Read the model definition and answer for the solid it produces. Units are mm, in the model's axes. A direction names the side the tool comes from. Give positions to 0.01 mm unless a question says otherwise; leave off trailing zeros. Loops run counter-clockwise (first coordinate to the right, second up) from the corner with the lowest first, then second, coordinate; pieces in that order, holes last.
(1) Which of the six approach directions +Z, -Z, +X, -X, +Y, -Y give full straight-line access (tool end or side, diameter ignored) to faces 1 (the face through (31.1, 9, 3)), 2 (the face through (47, 2.05, 6)), 3 (the face through (38, 5, 3.75)), 4 (the face through (59, 9.4, 6)), 5 (the face through (44.2, 4, 6))?
(2) Each of these flat-tipped pins is pushed along its axis until it touches: P1, Ø5, axis at x = 34.5, y = 8, coming from the -Z side; P2, Ø1.4, axis at x = 47, y = 3.5, coming from the +Z side; P3, Ø4.5, axis at x = 54.5, z = 8, coming from the +Y side; P4, Ø6, axis at y = 5, z = 6.5, coming from the -X side. Where does it stop, or does it pass through?
(3) Determine the mould class of faces 6 (the face through (39, 9, 5)), 7 (the face through (30, 8.9, -2)) for opening direction X: pulls with the +X half, pulls with the -X half, needs draft (parallel to the pull), parting line crosses it, or undercut.
(4) Straight lines are drawn through the part: probe 1 along X at (y, z) = (8.95, 6); probe 2 along X at (y, z) = (9.5, 3.75); probe 3 along Z at (x, y) = (32, 7.75). For each, find the intervals that lie inside material, in ascending order.
(5) Find section A-A, the plane x = 19. Write down the section's boundary in (y, z), then the cut area to 3 significant figures.
```python
from build123d import *
from build123d.topology import SkipClean

# Parameters (mm, degrees)
CROQUIS1_W              = 60.9
CROQUIS1_H              = 12
SALIENTE_EXTRUIR1_DEPTH = 14
CROQUIS2_OUTSIDE_W      = 75.626
CROQUIS2_OUTSIDE_H      = 26.726
CROQUIS2_OUTSIDE_R      = 1.5
CORTAR_EXTRUIR1_DEPTH   = 4
SALIENTE_EXTRUIR3_DEPTH = 1.1
CROQUIS4_OUTSIDE_W      = 75.752
CROQUIS4_OUTSIDE_H      = 29.852
CORTAR_EXTRUIR2_DEPTH   = 0.7
CORTAR_EXTRUIR3_DEPTH   = 2.5
CROQUIS6_W              = 1.45
CROQUIS6_H              = 3.1
CROQUIS6_W_2            = 1
CORTAR_EXTRUIR4_DEPTH   = 0.1
REDONDEO1_R             = 1
REDONDEO2_R             = 1
SALIENTE_EXTRUIR4_DEPTH = 0.1
CORTAR_EXTRUIR5_REACH   = 64.764
CROQUIS8_R              = 1.15
CROQUIS9_OUTSIDE_W      = 75.752
CROQUIS9_OUTSIDE_H      = 29.852
CORTAR_EXTRUIR7_DEPTH   = 5.55
SALIENTE_EXTRUIR6_DEPTH = 3.5
CROQUIS12_W             = 31.6
CROQUIS12_H             = 1.3
CORTAR_EXTRUIR8_DEPTH   = 2.3
CROQUIS14_W             = 1.3
CROQUIS14_H             = 1
CORTAR_EXTRUIR9_DEPTH   = 2.3
REDONDEO3_R             = 1
CROQUIS15_W             = 7.62
CROQUIS15_H             = 9.4
CROQUIS15_W_2           = 7.6
CORTAR_EXTRUIR10_DEPTH  = 1.9
REDONDEO4_R             = 1.3
REDONDEO5_R             = 1.3
REDONDEO6_R             = 1.3
REDONDEO7_R             = 1


# Some blends are built 0.0001 mm under size
with BuildPart() as part:
    # Croquis1 → Saliente-Extruir1 (new body)
    with BuildSketch(Plane(origin=(0, 0, 0), x_dir=(1, 0, 0), z_dir=(0, 1, 0))):
        with Locations((30.45, -6)):
            Rectangle(CROQUIS1_W, CROQUIS1_H)
    extrude(amount=SALIENTE_EXTRUIR1_DEPTH)

    # Croquis2 outside → Cortar-Extruir1 (cut)
    with BuildSketch(Plane(origin=(0, 14, 0), x_dir=(1, 0, 0), z_dir=(0, 1, 0))):
        with Locations((30.45, -6)):
            Rectangle(CROQUIS2_OUTSIDE_W, CROQUIS2_OUTSIDE_H)
        with Locations(Location((30.45, -6, 0), (0, 0, 270))):
            Circle(CROQUIS2_OUTSIDE_R, mode=Mode.SUBTRACT)
    extrude(amount=-CORTAR_EXTRUIR1_DEPTH, mode=Mode.SUBTRACT)

    # Croquis3 → Saliente-Extruir3 (add)
    with BuildSketch(Plane(origin=(0, 10, 0), x_dir=(1, 0, 0), z_dir=(0, 1, 0))):
        Polygon((30.45, 0), (29.45, 0), (29.45, 3), (31.45, 3), (31.45, 0), align=None)
    extrude(amount=-SALIENTE_EXTRUIR3_DEPTH)

    # Croquis4 outside → Cortar-Extruir2 (cut)
    with BuildSketch(Plane(origin=(0, 10, 0), x_dir=(1, 0, 0), z_dir=(0, 1, 0))):
        with Locations((30.45, -4.5)):
            Rectangle(CROQUIS4_OUTSIDE_W, CROQUIS4_OUTSIDE_H)
        Polygon((8.9, -6), (8.9, 0), (29.45, 0), (29.45, 3), (31.45, 3), (31.45, 0), (52, 0), (52, -12), (8.9, -12), align=None, mode=Mode.SUBTRACT)
    extrude(amount=-CORTAR_EXTRUIR2_DEPTH, mode=Mode.SUBTRACT)

    # Croquis5 → Cortar-Extruir3 (cut)
    with SkipClean():  # the faces are left unmerged after this step: merging them gives an invalid solid
        with BuildSketch(Plane(origin=(0, 10, 0), x_dir=(1, 0, 0), z_dir=(0, 1, 0))):
            with BuildLine():
                ThreePointArc((29.331966011, -5), (29.548647819, -4.801015327), (29.8, -4.648149417))
                Line((29.8, -4.648149417), (29.8, -1.9))
                Line((29.8, -1.9), (11.4, -1.9))
                Line((11.4, -1.9), (11.4, -5))
                Line((11.4, -5), (29.331966011, -5))
            make_face()
            with BuildLine():
                ThreePointArc((29.8, -7.351850583), (29.548647819, -7.198984673), (29.331966011, -7))
                Line((29.331966011, -7), (11.4, -7))
                Line((11.4, -7), (11.4, -10.1))
                Line((11.4, -10.1), (29.8, -10.1))
                Line((29.8, -10.1), (29.8, -7.351850583))
            make_face()
            with BuildLine():
                Line((49.05, -7), (31.568033989, -7))
                ThreePointArc((31.568033989, -7), (31.351352181, -7.198984673), (31.1, -7.351850583))
                Line((31.1, -7.351850583), (31.1, -10.1))
                Line((31.1, -10.1), (49.05, -10.1))
                Line((49.05, -10.1), (49.05, -7))
            make_face()
            with BuildLine():
                Line((49.05, -5), (49.05, -1.9))
                Line((49.05, -1.9), (31.1, -1.9))
                Line((31.1, -1.9), (31.1, -4.648149417))
                ThreePointArc((31.1, -4.648149417), (31.351352181, -4.801015327), (31.568033989, -5))
                Line((31.568033989, -5), (49.05, -5))
            make_face()
        extrude(amount=-CORTAR_EXTRUIR3_DEPTH, mode=Mode.SUBTRACT)

    # Croquis6 → Cortar-Extruir4 (cut)
    with SkipClean():  # the faces are left unmerged after this step: merging them gives an invalid solid
        with BuildSketch(Plane(origin=(0, 10, 0), x_dir=(1, 0, 0), z_dir=(0, 1, 0))):
            with Locations((49.775, -3.45)):
                Rectangle(CROQUIS6_W, CROQUIS6_H)
            with Locations((49.55, -8.55)):
                Rectangle(CROQUIS6_W_2, CROQUIS6_H)
            with Locations((10.9, -3.45)):
                Rectangle(CROQUIS6_W_2, CROQUIS6_H)
            with Locations((10.9, -8.55)):
                Rectangle(CROQUIS6_W_2, CROQUIS6_H)
        extrude(amount=-CORTAR_EXTRUIR4_DEPTH, mode=Mode.SUBTRACT)

    # Redondeo1
    redondeo1_edges = [part.edges().sort_by_distance(p)[0] for p in [
        (31.45, 9.45, -3),
    ]]
    fillet(redondeo1_edges, radius=REDONDEO1_R)

    # Redondeo2
    redondeo2_edges = [part.edges().sort_by_distance(p)[0] for p in [
        (29.45, 9.45, -3),
    ]]
    fillet(redondeo2_edges, radius=REDONDEO2_R - 0.0001)  # a hair under: the kernel refuses the full size

    # Croquis7 → Saliente-Extruir4 (add)
    with BuildSketch(Plane(origin=(0, 9.3, 0), x_dir=(1, 0, 0), z_dir=(0, 1, 0))):
        with BuildLine():
            Line((57.45, -8.8), (57.45, -7.15))
            ThreePointArc((57.45, -7.15), (58.6, -6), (57.45, -4.85))
            Line((57.45, -4.85), (57.45, -3.2))
            ThreePointArc((57.45, -3.2), (60.25, -6), (57.45, -8.8))
        make_face()
        with BuildLine():
            Line((3.75, -4.85), (3.75, -3.2))
            ThreePointArc((3.75, -3.2), (0.95, -6), (3.75, -8.8))
            Line((3.75, -8.8), (3.75, -7.15))
            ThreePointArc((3.75, -7.15), (2.6, -6), (3.75, -4.85))
        make_face()
    extrude(amount=SALIENTE_EXTRUIR4_DEPTH)

    # Croquis8 → Cortar-Extruir5 (cut, up to next)
    with BuildSketch(Plane(origin=(0, 9.3, 0), x_dir=(1, 0, 0), z_dir=(0, 1, 0)), mode=Mode.PRIVATE) as cortar_extruir5_sk1:
        with Locations(Location((57.45, -6, 0), (0, 0, 90))):
            Circle(CROQUIS8_R)
    cortar_extruir5_tool1 = extrude(cortar_extruir5_sk1.sketch, amount=-CORTAR_EXTRUIR5_REACH, mode=Mode.PRIVATE) & part.part
    # Croquis8 → Cortar-Extruir5 (cut, up to next)
    with BuildSketch(Plane(origin=(0, 9.3, 0), x_dir=(1, 0, 0), z_dir=(0, 1, 0)), mode=Mode.PRIVATE) as cortar_extruir5_sk2:
        with Locations(Location((3.75, -6, 0), (0, 0, 90))):
            Circle(CROQUIS8_R)
    cortar_extruir5_tool2 = extrude(cortar_extruir5_sk2.sketch, amount=-CORTAR_EXTRUIR5_REACH, mode=Mode.PRIVATE) & part.part
    add(cortar_extruir5_tool1.solids().sort_by_distance((57.45, 9.3, 6))[0], mode=Mode.SUBTRACT)
    add(cortar_extruir5_tool2.solids().sort_by_distance((3.75, 9.3, 6))[0], mode=Mode.SUBTRACT)

    # Croquis9 outside → Cortar-Extruir7 (cut)
    with BuildSketch(Plane.XZ):
        with Locations((30.45, 4.5)):
            Rectangle(CROQUIS9_OUTSIDE_W, CROQUIS9_OUTSIDE_H)
        Polygon((30, 7.25), (28.1, 7.25), (28.1, 4.75), (31.9, 4.75), (31.9, 7.25), align=None, mode=Mode.SUBTRACT)
    extrude(amount=-CORTAR_EXTRUIR7_DEPTH, mode=Mode.SUBTRACT)

    # Croquis10 → Saliente-Extruir6 (add)
    with BuildSketch(Plane.XZ.offset(-5.55)):
        Polygon((30.65, 4.75), (29.35, 4.75), (29.35, 3.75), (14.2, 3.75), (14.2, 5.34), (15.8, 5.34), (15.8, 5.95), (15.8, 6.56), (14.2, 6.56), (14.2, 9.45), (12.5, 9.45), (12.5, 2.45), (29.35, 2.45), (30, 2.45), (30.65, 2.45), (47.5, 2.45), (47.5, 9.45), (45.8, 9.45), (45.8, 6.56), (44.2, 6.56), (44.2, 5.95), (44.2, 5.34), (45.8, 5.34), (45.8, 3.75), (30.65, 3.75), align=None)
    extrude(amount=SALIENTE_EXTRUIR6_DEPTH)

    # Croquis12 → Cortar-Extruir8 (cut)
    with BuildSketch(Plane.XZ.offset(-2.05)):
        with Locations((30, 3.1)):
            Rectangle(CROQUIS12_W, CROQUIS12_H)
    extrude(amount=-CORTAR_EXTRUIR8_DEPTH, mode=Mode.SUBTRACT)

    # Croquis14 → Cortar-Extruir9 (cut)
    with BuildSketch(Plane.XZ.offset(-2.05)):
        with Locations((30, 4.25)):
            Rectangle(CROQUIS14_W, CROQUIS14_H)
    extrude(amount=-CORTAR_EXTRUIR9_DEPTH, mode=Mode.SUBTRACT)

    # Redondeo3
    # the kernel refuses this fillet: 1 mm, written as the material it adds along each edge
    with BuildSketch(Plane(origin=(29.35, 4.35, 4.75), x_dir=(0, -1, 0), z_dir=(1, 0, 0))) as redondeo3_piece_1:
        with BuildLine():
            CenterArc((REDONDEO3_R, REDONDEO3_R), REDONDEO3_R, 180, 90)
            Line((0, REDONDEO3_R), (0, 0))
            Line((0, 0), (REDONDEO3_R, 0))
        make_face()
    extrude(amount=1.3)

    # Croquis15 → Cortar-Extruir10 (cut)
    with BuildSketch(Plane.XZ.offset(-5.55)):
        with Locations((55.79, 6)):
            Rectangle(CROQUIS15_W, CROQUIS15_H)
        with Locations((5.1, 6)):
            Rectangle(CROQUIS15_W_2, CROQUIS15_H)
    extrude(amount=-CORTAR_EXTRUIR10_DEPTH, mode=Mode.SUBTRACT)

    # Redondeo4
    redondeo4_edges = [part.edges().sort_by_distance(p)[0] for p in [
        (60.9, 7.425, 0),
    ]]
    fillet(redondeo4_edges, radius=REDONDEO4_R)

    # Redondeo5
    redondeo5_edges = [part.edges().sort_by_distance(p)[0] for p in [
        (60.9, 7.425, 12),
        (0, 7.425, 12),
        (0, 7.425, 0),
    ]]
    fillet(redondeo5_edges, radius=REDONDEO5_R)

    # Redondeo6
    redondeo6_edges = [part.edges().sort_by_distance(p)[0] for p in [
        (59.6, 6.5, 10.7),
        (59.6, 6.5, 1.3),
        (1.3, 6.5, 1.3),
        (1.3, 6.5, 10.7),
    ]]
    fillet(redondeo6_edges, radius=REDONDEO6_R)

    # Redondeo7
    redondeo7_edges = [part.edges().sort_by_distance(p)[0] for p in [
        (31.9, 2.775, 4.75),
        (28.1, 2.775, 4.75),
        (28.1, 2.775, 7.25),
        (31.9, 2.775, 7.25),
    ]]
    fillet(redondeo7_edges, radius=REDONDEO7_R)


solid = part.part
```
Entries:
1. face 1: +Y
1. face 2: +Z, -Z, +X, -Y
1. face 3: -Y
1. face 4: +Z, -Z, +X, +Y
1. face 5: +Z, -Y
2. P1: stops at z = 0
2. P2: stops at z = 9.45
2. P3: stops at y = 9.3
2. P4: stops at x = 0
3. face 6: undercut
3. face 7: needs draft
4. probe 1: x = 0 to 2.6, 4.9 to 56.3, 58.6 to 60.9
4. probe 2: x = 8.9 to 11.4, 29.8 to 31.1, 49.05 to 52
4. probe 3: z = 0 to 1.9, 5 to 7, 10.1 to 12
5. outline: (4.35, 2.45) - (5.55, 2.45) - (5.55, 0) - (10, 0) - (10, 1.9) - (7.5, 1.9) - (7.5, 5) - (10, 5) - (10, 7) - (7.5, 7) - (7.5, 10.1) - (10, 10.1) - (10, 12) - (5.55, 12) - (5.55, 3.75) - (4.35, 3.75) - close
5. area: 39.5 mm2
